Could you check a few things on this model? Use its own coordinates, in mm. Coordinates: 2 decimals unless noted, no trailing zeros. Write each loop counter-clockwise with the first axis right and the second up, starting at its lowest first coordinate (ties: lowest second). Pieces come first, ordered by that corner, then holes. Notation, with made-up numbers: (20.25, -2.5) - (35.25, -2.5) arc R33 cw to (35.25, 35.5) - close; hole circle Ø8 at (31.5, 9). An arc over 180 degrees is marked (long way). Write item = value, one per line. Start each with the question number.
```python
from build123d import *

# Parameters (mm, degrees)
SKETCH1_R           = 3.175
BOSS_EXTRUDE1_DEPTH = 6.35
SKETCH2_W           = 168.075192403
SKETCH2_H           = 32.004
BOSS_EXTRUDE2_DEPTH = 12.7
SKETCH5_R           = 3.175
BOSS_EXTRUDE3_DEPTH = 6.35
SKETCH7_W           = 12.7
SKETCH7_H           = 32.004
CUT_EXTRUDE1_DEPTH  = 10.16


with BuildPart() as part:
    # Sketch1 → Boss-Extrude1 (new body)
    with BuildSketch(Plane.XY):
        with BuildLine():
            Line((-47.217391304, 7.923913043), (155.982608696, 7.923913043))
            ThreePointArc((155.982608696, 7.923913043), (171.984608696, -8.078086957), (155.982608696, -24.080086957))
            Line((155.982608696, -24.080086957), (-47.217391304, -24.080086957))
            ThreePointArc((-47.217391304, -24.080086957), (-63.219391304, -8.078086957), (-47.217391304, 7.923913043))
        make_face()
        with Locations((-47.217391304, -8.078086957)):
            Circle(SKETCH1_R, mode=Mode.SUBTRACT)
        with Locations((155.982608696, -8.078086957)):
            Circle(SKETCH1_R, mode=Mode.SUBTRACT)
    extrude(amount=BOSS_EXTRUDE1_DEPTH)

    # Sketch2 → Boss-Extrude2 (add)
    with BuildSketch(Plane.XY.offset(6.35)):
        with Locations((54.045012495, -8.078086957)):
            Rectangle(SKETCH2_W, SKETCH2_H)
    extrude(amount=BOSS_EXTRUDE2_DEPTH)

    # Sketch5 → Boss-Extrude3 (add)
    with BuildSketch(Plane.XY.offset(19.05)):
        with BuildLine():
            Line((-47.217391304, 7.923913043), (155.982608696, 7.923913043))
            ThreePointArc((155.982608696, 7.923913043), (171.984608696, -8.078086957), (155.982608696, -24.080086957))
            Line((155.982608696, -24.080086957), (-47.217391304, -24.080086957))
            ThreePointArc((-47.217391304, -24.080086957), (-63.219391304, -8.078086957), (-47.217391304, 7.923913043))
        make_face()
        with Locations((-47.217391304, -8.078086957)):
            Circle(SKETCH5_R, mode=Mode.SUBTRACT)
        with Locations((155.982608696, -8.078086957)):
            Circle(SKETCH5_R, mode=Mode.SUBTRACT)
    extrude(amount=BOSS_EXTRUDE3_DEPTH)

    # Sketch7 → Cut-Extrude1 (cut)
    with BuildSketch(Plane.ZY.offset(29.992583707)):
        with Locations((12.7, -8.078086957)):
            Rectangle(SKETCH7_W, SKETCH7_H)
    extrude(amount=-CUT_EXTRUDE1_DEPTH, mode=Mode.SUBTRACT)


solid = part.part
```
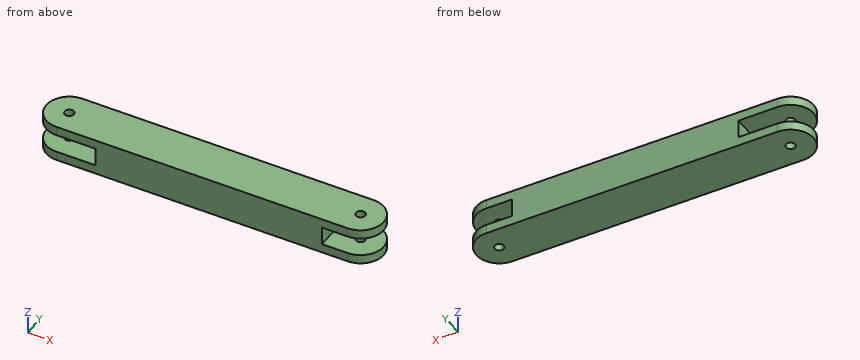
1) If I drill on probe 1 along Z at (x, y) = (152.5, -17.5); probe 2 along X at (y, z) = (-9, 21.5); probe 3 along X at (y, z) = (-18.5, 10), over which ranges is the centre line in solid material (lowest first)? Write a range as [from, to].
2) Suppose I cut it at A-A on x = -33. Please give me the cut outline in (y, z), plus the area to 3 significant figures.
3) Suppose I cut it at D-D on z = 11.75. Please give me the cut outline in (x, y), plus the area to 3 significant figures.
4) For P1, Ø4, axis at y = -19.5, z = 3, coming from the +X side; P2, Ø4, axis at x = 155.98, y = -8.08, coming from the +Z side; P3, Ø4, axis at y = -3.5, z = 10, coming from the -X side, each with a flat end and sliding along its axis, tell me the tip position at first contact or that it passes through.
5) Suppose I cut it at C-C on z = 22.75. Please give me the cut outline in (x, y) (3 decimals), plus the area to 3 significant figures.
6) Suppose I cut it at B-B on y = -16. Please give me the cut outline in (x, z).
Reply:
q1.probe_1 = [0, 6.35], [19.05, 25.4]
q1.probe_2 = [-63.19, -50.26], [-44.18, 152.94], [159.02, 171.96]
q1.probe_3 = [-19.83, 138.08]
q2.outline = (-24.08, 0) - (7.92, 0) - (7.92, 6.35) - (-24.08, 6.35) - close; (-24.08, 19.05) - (7.92, 19.05) - (7.92, 25.4) - (-24.08, 25.4) - close
q2.area = 406 mm^2
q3.outline = (-19.83, -24.08) - (138.08, -24.08) - (138.08, 7.92) - (-19.83, 7.92) - close
q3.area = 5,050 mm^2
q4.P1 = 168.92
q4.P2 = through
q4.P3 = -19.83
q5.outline = (-47.217, -24.08) - (155.983, -24.08) arc R16.002 ccw to (155.983, 7.924) - (-47.217, 7.924) arc R16.002 ccw to start; hole circle Ø6.35 at (-47.217, -8.078); hole circle Ø6.35 at (155.983, -8.078)
q5.area = 7,240 mm^2
q6.outline = (-61.12, 0) - (169.89, 0) - (169.89, 6.35) - (138.08, 6.35) - (138.08, 19.05) - (169.89, 19.05) - (169.89, 25.4) - (-61.12, 25.4) - (-61.12, 19.05) - (-19.83, 19.05) - (-19.83, 6.35) - (-61.12, 6.35) - close
